CAD build for the part. Positions are in the model's coordinates, mm. A direction names the side the tool comes from. Give positions to 0.01 mm unless a question says otherwise; leave off trailing zeros. Write each loop counter-clockwise with the first axis right and the second up, starting at its lowest first coordinate (ties: lowest second). Pieces come first, ordered by that corner, then holes. Notation, with made-up numbers: (10.5, 59.25) - (52.5, 59.25) arc R21 cw to (52.5, 73.25) - close; hole circle Ø11 at (82, -25). An arc over 180 degrees is marked (long way). Put each result on its own line as item: value. Start each with the question number.
1. Cut at A-A on x = 4.75. List the corners of the cut face in (y, z), and give its area (3 significant figures).
2. Tool access for faces 1 (the cylindrical face through (4.61, -0.33, 1.04)), 2 (the cylindrical face through (1.21, 2.07, -0.46)): list every direction of +Z, -Z, +X, -X, +Y, -Y with a clear straight run to the whole face (end or side of a thin tool).
3. Wall check: line 1 (Y direction, x = 3.5, z = 0); line 2 (Z direction, x = 1.25, y = 0.1); line 3 (Y direction, x = 0.5, z = 0.1). Give the ranges that are in metal, low to high.
4. Drop flat-ended pins along their axis: pin 1 (1.5 mm diameter, centred on x = 5.5, z = -1.5, fed in from -Y); pin 2 (1.5 mm diameter, centred on x = 3, y = -1.5, fed in from -Z). Give the stop position or say it passes through.
from build123d import *

# Parameters (mm, degrees)
CIRPATTERN1_COUNT = 2
CIRPATTERN1_ANGLE = 90
CHAMFER1_SIZE     = 0.2032


with BuildPart() as part:
    # BodySke → Base-Revolve (revolve)
    with BuildSketch(Plane.XY, mode=Mode.PRIVATE) as base_revolve_sk:
        with BuildLine():
            Line((1.5748, 1.0922), (1.5748, 2.1209))
            Line((1.5748, 2.1209), (0.845695803, 2.1209))
            ThreePointArc((0.845695803, 2.1209), (0.728748015, 2.09237553), (0.638066948, 2.013208777))
            ThreePointArc((0.638066948, 2.013208777), (0.163333253, 1.05595206), (0, 0))
            Line((0, 0), (7.9248, 0))
            Line((7.9248, 0), (7.9248, 1.0922))
            Line((7.9248, 1.0922), (1.5748, 1.0922))
        make_face()
    revolve(base_revolve_sk.sketch.rotate(Axis((-25.4, 0, 0), (1, 0, 0)), 90), axis=Axis((-25.4, 0, 0), (1, 0, 0)))

    # Sketch3 → Cut-Loft1 section 0
    with BuildSketch(Plane(origin=(0, 0, 0), x_dir=(0, 0, -1), z_dir=(1, 0, 0))):
        with BuildLine():
            Line((0.3429, -1.3843), (-0.3429, -1.3843))
            Line((-0.3429, -1.3843), (-0.3429, 1.3843))
            Line((-0.3429, 1.3843), (0.3429, 1.3843))
            Line((0.3429, 1.3843), (0.3429, -1.3843))
        make_face()
    # Sketch4 → Cut-Loft1 section 1
    with BuildSketch(Plane(origin=(1.4986, 0, 0), x_dir=(0, 0, -1), z_dir=(1, 0, 0))):
        with BuildLine():
            Line((0.17145, -0.17145), (-0.17145, -0.17145))
            Line((-0.17145, -0.17145), (-0.17145, 0.17145))
            Line((-0.17145, 0.17145), (0.17145, 0.17145))
            Line((0.17145, 0.17145), (0.17145, -0.17145))
        make_face()
    cut_loft1 = loft(mode=Mode.SUBTRACT)

    # CirPattern1: Cut-Loft1 ×2 about axis
    cirpattern1_axis = Axis((0, 0, 0), (1, 0, 0))
    for i in range(1, CIRPATTERN1_COUNT):
        add(cut_loft1.rotate(cirpattern1_axis, i * CIRPATTERN1_ANGLE / (CIRPATTERN1_COUNT - 1)), mode=Mode.SUBTRACT)

    # Chamfer1
    chamfer1_edges = [part.edges().sort_by_distance(p)[0] for p in [
        (7.9248, 0, -1.0922),
    ]]
    chamfer(chamfer1_edges, length=CHAMFER1_SIZE)


solid = part.part
Report:
1. outline: circle Ø2.18 at (0, 0)
1. area: 3.75 mm²
2. face 1: +X
2. face 2: +X, -X
3. line 1: y = -1.09 to 1.09
3. line 2: z = -2.12 to -0.37, 0.37 to 2.12
3. line 3: y = -1.8 to -0.98, 0.98 to 1.8
4. pin 1: stops at y = -0.79
4. pin 2: stops at z = -0.79
